Input: part model. Units: mm. Frame: model coordinates. A direction names the side the tool comes from. Give positions to 0.01 mm unless a question says otherwise; leave off trailing zeros. Loops run counter-clockwise (first coordinate to the right, second up) from the corner with the lowest first, then second, coordinate; pieces in that order, holes last. Notation, with made-up numbers: M 22,2 L 47,2 A9 ccw 47,12 Z; hole C 21.25,81 d1. An arc over 180 degrees is marked long. Answer as a JSON object with one key per item and string values. Group by question number.
Autodesk Inventor part; units mm, degrees
ref_plane "Work Plane1" through (0, 0, 0) normal (0, 0, 1) x (1, 0, 0)
ref_plane "YZ Plane" through (0, 0, 0) normal (1, 0, 0) x (0, 1, 0)
ref_plane "XZ Plane" through (0, 0, 0) normal (0, 1, 0) x (-1, 0, 0)
ref_plane "Work Plane1" through (0, 0, 0) normal (0, 0, 1) x (1, 0, 0)
sketch "Sketch1" plane through (0, 0, 0) normal (0, 0, 1) x (1, 0, 0)
  circle A0 centre (39.1667, -0.7223) radius 5
  circle A1 centre (-39.1667, -0.7223) radius 5
  line L0 (-50, -13) -> (-28.3333, -13)
  line L1 (-28.3333, -13) -> (-28.3333, 10)
  line L2 (-28.3333, 10) -> (28.3333, 10)
  line L3 (28.3333, -13) -> (28.3333, 10)
  line L4 (28.3333, -13) -> (50, -13)
  line L5 (50, -13) -> (50, 13)
  line L6 (50, 13) -> (-50, 13)
  line L7 (-50, 13) -> (-50, -13)
  line L8 (28.3333, -161) -> (31.3333, -161)
  line L9 (31.3333, -161) -> (31.3333, -13)
  line L10 (31.3333, -13) -> (28.3333, -13)
  line L11 (28.3333, -13) -> (28.3333, -161)
  circle A2 centre (39.1667, -173.2777) radius 5
  circle A3 centre (-39.1667, -173.2777) radius 5
  line L12 (50, -161) -> (28.3333, -161)
  line L13 (28.3333, -161) -> (28.3333, -184)
  line L14 (28.3333, -184) -> (-28.3333, -184)
  line L15 (-28.3333, -161) -> (-28.3333, -184)
  line L16 (-28.3333, -161) -> (-50, -161)
  line L17 (-50, -161) -> (-50, -187)
  line L18 (-50, -187) -> (50, -187)
  line L19 (50, -187) -> (50, -161)
  line L20 (-31.3333, -161) -> (-28.3333, -161)
  line L21 (-28.3333, -161) -> (-28.3333, -13)
  line L22 (-28.3333, -13) -> (-31.3333, -13)
  line L23 (-31.3333, -13) -> (-31.3333, -161)
  line L24 (-31.3333, -161) -> (-28.3333, -161)
  line L25 (-28.3333, -161) -> (-28.3333, -13)
  line L26 (-28.3333, -13) -> (-31.3333, -13)
  line L27 (-31.3333, -13) -> (-31.3333, -161)
  line L28 (53, 16) -> (-53, 16)
  line L29 (-53, 16) -> (-53, -187)
  line L30 (53, -187) -> (53, 16)
  line L31 (53, 16) -> (-53, -187) construction
  line L32 (-53, 16) -> (53, -187) construction
  line L33 (53, -187) -> (53, -190)
  line L34 (53, -190) -> (-53, -190)
  line L35 (-53, -190) -> (-53, -187)
  point P0 (0, 0)
  point P1 (0, -85.5)
  dimension "d0" = 106
  dimension "d1" = 203
  dimension "d2" = 3
extrude "Extrusion1" add sketch "Sketch1" along normal blind 5 contours L7 L6 L5 L4 L3 L2 L1 L0 | L0 L21 L16 L23 | L1 L2 L3 L11 L13 L14 L15 L21 | L16 L15 L14 L13 L8 L12 L19 L18 L17 | L9 L8 L11 L4 | L30 L33 L34 L35 L29 L28
sketch "Sketch2" plane through (0, 0, 0) normal (0, 0, -1) x (-1, 0, 0)
  line L0 (-53, 16) -> (53, 16)
  line L1 (-53, -190) -> (-53, 16)
  line L2 (53, -190) -> (-53, -190)
  line L3 (53, 16) -> (53, -190)
  line L4 (-50, 13) -> (50, 13)
  line L5 (50, 13) -> (50, -187)
  line L6 (50, -187) -> (-50, -187)
  line L7 (-50, -187) -> (-50, 13)
  point P0 (0, 0)
  dimension "d5" = 3
extrude "Extrusion2" add sketch "Sketch2" along normal blind 15
sketch "Sketch3" plane through (53, -190, 5) normal (1, 0, 0) x (0, 0, -1)
  line L0 (0, 206) -> (20, 206)
  line L1 (0, 0) -> (0, 206)
  line L2 (20, 0) -> (0, 0)
  line L3 (20, 206) -> (20, 0)
  point P0 (5, 190)
sketch "Sketch4" plane through (53, -190, 5) normal (1, 0, 0) x (0, 0, -1)
  line L0 (0, 0) -> (0, 206)
  line L1 (20, 206) -> (20, 0)
  line L2 (5, 177) -> (58, 177)
  line L3 (20, 177) -> (0, 177)
  line L4 (58, 29) -> (5, 29)
  line L5 (20, 29) -> (0, 29)
  line L6 (12.6827, 177) -> (12.6827, 29)
  point P0 (5, 190)
extrude "Extrusion3" cut sketch "Sketch4" against normal up to surface (106 mm away) contours L6 L2 L1 L4
properties part number "bawah"
1. Mould query, pull axis X, two halves, no side actions, for faces 3 (the flat face through (0, -188, -15)), 4 (the flat face through (53, -88, -3)), 5 (the flat face through (-50, -86, -6)). Classes: pulls with the +X half, pulls with the -X half, needs draft (parallel to the pull), parting line crosses it, or undercut.
2. Reachability of faces 1 (the flat face through (50, -88, -6)), 2 (the flat face through (0.2, 13.4, -15)) from +Z, -Z, +X, -X, +Y, -Y: full face, straight path, thin tool, end or side. Return the list, or none.
3. Section A-A (z = -4.5). Output: boundary loops of the cut face in (x, y).
4. Material intervals for L1, parallel to X at y = -146, z = -6.25; L2, parallel to Y at x = 37.5, z = 0.5; L3, parallel to Y at x = 19, z = -2.75, sorted ascending.
5. First-contact query: P1, Ø3.5, axis at x = 51, y = -108.5, coming from the -Z side; P2, Ø6, axis at x = -39.17, y = -173.28, coming from the -Z side; P3, Ø1.5, axis at x = -31.5, y = -109, coming from the -Z side. Flat tips, straight axial feed; report the tip coordinate or a pass-through.
6. Section B-B (y = -67). Output: boundary loops of the cut face in (x, z).
7. Section D-D (x = 1). Output: boundary loops of the cut face in (y, z), then the cut area to 3 significant figures.
8. Section C-C (x = 37). Output: boundary loops of the cut face in (y, z), then the cut area to 3 significant figures.
Geometry results:
{
 "1": {"face 3": "needs draft", "face 4": "pulls with the +X half", "face 5": "undercut"},
 "2": {"face 1": "-Z", "face 2": "-Z, +X, -X, +Y, -Y"},
 "3": {"outline": "M -53,-190 L 53,-190 L 53,16 L -53,16 Z; hole M -50,-187 L 50,-187 L 50,13 L -50,13 Z"},
 "4": {"L1": "-53 to -50, 50 to 53", "L2": "-190 to -177.99, -168.56 to -5.44, 3.99 to 16", "L3": "-190 to -187, 13 to 16"},
 "5": {"P1": "z = -7.68", "P2": "through", "P3": "z = 0"},
 "6": {"outline": "M -53,-7.68 L -50,-7.68 L -50,0 L 50,0 L 50,-7.68 L 53,-7.68 L 53,5 L -53,5 Z"},
 "7": {"outline": "M -190,-15 L -187,-15 L -187,0 L 13,0 L 13,-15 L 16,-15 L 16,5 L -190,5 Z", "area": "1,120 mm2"},
 "8": {"outline": "M -190,-15 L -187,-15 L -187,0 L -177.78,0 L -177.78,5 L -190,5 Z; M -168.77,0 L -5.23,0 L -5.23,5 L -168.77,5 Z; M 3.78,0 L 13,0 L 13,-15 L 16,-15 L 16,5 L 3.78,5 Z", "area": "1,030 mm2"}
}
